from build123d import *

# Parameters (mm, degrees)
F1_DEPTH = 6.35


with BuildPart() as f1:
    # F0 (on Top) → F1 (new body)
    with BuildSketch(Plane.XY):
        with BuildLine():
            ThreePointArc((-3.175, 0), (-2.2450640303, 2.2450640303), (0, 3.175))
            Line((0, 3.175), (0, 9.525))
            ThreePointArc((0, 9.525), (-6.7351920908, 6.7351920908), (-9.525, 0))
            Line((-9.5250000075, 0), (-3.175, 0))
        make_face()
        with BuildLine():
            Line((0, 9.525), (0, 3.175))
            ThreePointArc((0, 3.175), (2.2450640303, 2.2450640303), (3.175, 0))
            Line((3.175, 0), (9.525, 0))
            ThreePointArc((9.525, 0), (6.7351920908, 6.7351920908), (0, 9.525))
        make_face()
        with BuildLine():
            Line((9.525, 0), (3.175, 0))
            ThreePointArc((3.175, 0), (0, -3.175), (-3.175, 0))
            Line((-3.175, 0), (-9.5250000075, 0))
            ThreePointArc((-9.525, 0), (0, -9.525), (9.525, 0))
        make_face()
        with BuildLine():
            ThreePointArc((-9.525, 0), (-6.7351920908, 6.7351920908), (0, 9.525))
            Line((0, 9.525), (0, 45.4219387724))
            ThreePointArc((0, 45.4219387724), (-6.6627997611, 48.1401242205), (-9.5228225449, 54.7432827422))
            Line((-9.5228225449, 54.7432827422), (-9.5250000075, 0))
        make_face()
        with BuildLine():
            Line((0, 45.4219387724), (0, 9.525))
            ThreePointArc((0, 9.525), (6.7351920908, 6.7351920908), (9.525, 0))
            Line((9.525, 0), (9.525, 54.9469387724))
            ThreePointArc((9.525, 54.9469387724), (6.7351920908, 48.2117466816), (0, 45.4219387724))
        make_face()
        with BuildLine():
            ThreePointArc((-9.5228225449, 54.7432827422), (-6.6627997611, 48.1401242205), (0, 45.4219387724))
            ThreePointArc((0, 45.4219387724), (6.7351920908, 48.2117466816), (9.525, 54.9469387724))
            ThreePointArc((9.525, 54.9469387724), (-0.1018338352, 64.4713943931), (-9.5228225449, 54.7432827422))
        make_face()
        with BuildLine():
            ThreePointArc((3.175, 54.9469387724), (2.2450640303, 52.7018747421), (0, 51.7719387724))
            ThreePointArc((0, 51.7719387724), (-2.2450640303, 57.1920028027), (3.175, 54.9469387724))
        make_face(mode=Mode.SUBTRACT)
    extrude(amount=F1_DEPTH)


solid = f1.part
The model under review builds one solid part; all positions refer to its coordinate system, in mm. Coordinates: 2 decimals unless noted, no trailing zeros. Loops run counter-clockwise (first coordinate to the right, second up) from the corner with the lowest first, then second, coordinate; pieces in that order, holes last. Notation, with made-up numbers: M -25.5,-33 L 22.5,-33 A8 cw 22.5,-21 Z; hole C 14.25,29 d4. An arc over 180 degrees is marked long. Put each result on its own line as item: value. Start each with the question number.
Q1. Add section D-D (x = 5). Write out the cut boundary in (y, z).
Q2. Add section A-A (z = 4). Write out the cut boundary in (x, y) (3 decimals), and give its area (3 significant figures).
Q3. Add section B-B (x = 0.75). Write out the cut boundary in (y, z).
Q4. Wall thickness on line 1 (Y direction, x = 0, z = 2.5) (3 decimals); line 2 (Y direction, x = -2.5, z = 4.5); line 3 (X direction, y = 41, z = 5.75) (3 decimals): over which ranges is each line inside the solid? List them lowest first.
Q5. Add section C-C (y = -1). Write out the cut boundary in (x, z).
Answers:
1. outline: M -8.11,0 L 63.05,0 L 63.05,6.35 L -8.11,6.35 Z
2. outline: M -9.525,0 A9.525 ccw 9.525,0 L 9.525,54.947 A9.525 ccw long -9.523,54.743 Z; hole C 0,0 d6.35; hole C 0,54.947 d6.35
2. area: 1,270 mm^2
3. outline: M -9.5,0 L -3.09,0 L -3.09,6.35 L -9.5,6.35 Z; M 3.09,0 L 51.86,0 L 51.86,6.35 L 3.09,6.35 Z; M 58.03,0 L 64.44,0 L 64.44,6.35 L 58.03,6.35 Z
4. line 1: y = -9.525 to -3.175, 3.175 to 51.772, 58.122 to 64.472
4. line 2: y = -9.19 to -1.96, 1.96 to 52.99, 56.9 to 64.14
4. line 3: x = -9.523 to 9.525
5. outline: M -9.47,0 L -3.01,0 L -3.01,6.35 L -9.47,6.35 Z; M 3.01,0 L 9.47,0 L 9.47,6.35 L 3.01,6.35 Z
